```python
from build123d import *

# Parameters (mm, degrees)
F1_DEPTH = 20
F2_R     = 2


with BuildPart() as f1:
    # F0 (on Front) → F1 (new body)
    with BuildSketch(Plane.XZ):
        Polygon((-19.228746, -9.445448), (0.771254, -9.445448), (0.771254, 0.554552), (-9.228746, 10.554552), (-19.228746, 10.554552), align=None)
    extrude(amount=F1_DEPTH)

    # F2
    f2_edges = [f1.edges().sort_by_distance(p)[0] for p in [
        (-14.228746, 0, 10.554552),
        (-14.228746, -20, 10.554552),
    ]]
    fillet(f2_edges, radius=F2_R)


solid = f1.part
```
Here's how the part is built. I have some questions about the finished solid (model axes, mm). Coordinates: 2 decimals unless noted, no trailing zeros. Order: outer loops, then holes, each group sorted by start corner. A loop starts at its lowest first (then second) coordinate and runs counter-clockwise, first axis right, second up. Notation, with made-up numbers: (-33, 36) -> (-12, 36) arc R29 cw to (-12, 66) -> close; hole circle Ø10 at (78.25, 33). An arc over 180 degrees is marked (long way). Return JSON: item names as keys, results as strings.
1) If we section it at A-A on y = -11: List the corners of the cut face in (x, z) for me.
Conclusion:
{"outline": "(-19.23, -9.45) -> (0.77, -9.45) -> (0.77, 0.55) -> (-9.23, 10.55) -> (-19.23, 10.55) -> close"}
2) If I drill on probe 1 along X at (y, z) = (-12, 6.25); probe 2 along Z at (x, y) = (-11, -1.25); probe 3 along X at (y, z) = (-7, 9.5), over which ranges is the centre line in solid material (lowest first)?
Conclusion:
{"probe 1": "x = -19.23 to -4.92", "probe 2": "z = -9.45 to 10.41", "probe 3": "x = -19.23 to -8.17"}
3) I'm going to push a flat-ended pin straight in: P1, Ø3, axis at x = -10, z = -5, coming from the +Y side. Where does the tip first touch, or does it pass through?
Conclusion:
{"P1": "stops at y = 0"}
4) If we section it at B-B on z = 9.5: List the corners of the cut face in (x, y) for me.
Conclusion:
{"outline": "(-19.23, -19.76) -> (-8.17, -19.76) -> (-8.17, -0.24) -> (-19.23, -0.24) -> close"}
5) If we section it at C-C on x = -5: List the corners of the cut face in (y, z) for me.
Conclusion:
{"outline": "(-20, -9.45) -> (0, -9.45) -> (0, 6.33) -> (-20, 6.33) -> close"}
